from build123d import *

# Parameters (mm, degrees)
REVOLVE_THIN1_ANGLE = 60
SKETCH3_R           = 45
BOSS_EXTRUDE2_DEPTH = 648.5
SKETCH4_R           = 28
CUT_EXTRUDE1_DEPTH  = 40
CUT_EXTRUDE2_DEPTH  = 40


# Read off the part's stored shape, not the designer's step: Revolve-Thin1
with BuildPart() as part:
    # Revolve-Thin1 outline → Revolve-Thin1 (revolve)
    with BuildSketch(Plane(origin=(-45, 0, 0), x_dir=(1, 0, 0), z_dir=(0, 0, 1))):
        with BuildLine():
            Line((35, -19.5), (0, -19.5))
            Line((0, -19.5), (0, -29.5))
            Line((0, -29.5), (45, -29.5))
            Line((45, -29.5), (45, -9.5))
            ThreePointArc((45, -9.5), (54.5, 0), (45, 9.5))
            Line((45, 9.5), (45, 619))
            Line((45, 619), (0, 619))
            Line((0, 619), (0, 609))
            Line((0, 609), (35, 609))
            Line((35, 609), (35, -19.5))
        make_face()
    revolve(axis=Axis((-45, 0, 0), (0, 1, 0)), revolution_arc=REVOLVE_THIN1_ANGLE)

    # Sketch3 → Boss-Extrude2 (add)
    with BuildSketch(Plane(origin=(0, 619, 0), x_dir=(1, 0, 0), z_dir=(0, 1, 0))):
        with Locations(Location((-45, 0, 0), (0, 0, 90))):
            Circle(SKETCH3_R)
    extrude(amount=-BOSS_EXTRUDE2_DEPTH)

    # Sketch4 → Cut-Extrude1 (cut)
    with BuildSketch(Plane(origin=(0, 619, 0), x_dir=(1, 0, 0), z_dir=(0, 1, 0))):
        with Locations(Location((-45, 0, 0), (0, 0, 270))):
            Circle(SKETCH4_R)
    extrude(amount=-CUT_EXTRUDE1_DEPTH, mode=Mode.SUBTRACT)

    # Sketch5 → Cut-Extrude2 (cut)
    with BuildSketch(Plane(origin=(0, 619, 0), x_dir=(1, 0, 0), z_dir=(0, 1, 0))):
        with BuildLine():
            Line((-18.321356856, 8.5), (-12, 8.5))
            Line((-12, 8.5), (-12, -8.5))
            Line((-12, -8.5), (-18.321356856, -8.5))
            ThreePointArc((-18.321356856, -8.5), (-17, 0), (-18.321356856, 8.5))
        make_face()
    extrude(amount=-CUT_EXTRUDE2_DEPTH, mode=Mode.SUBTRACT)


solid = part.part
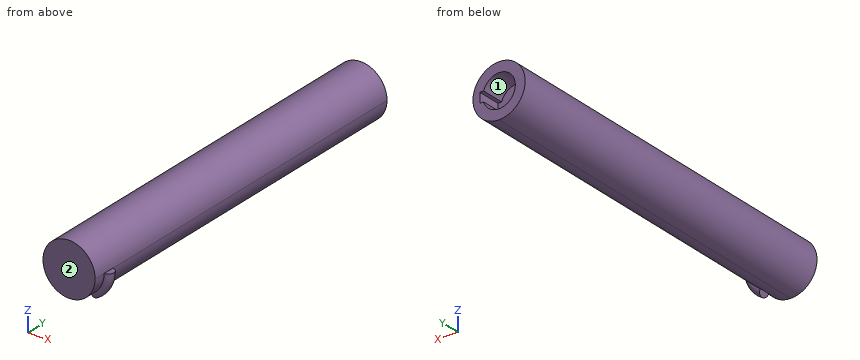
Input: part model. Units: mm. Frame: model coordinates. Face numbers are marked on the shaded views. Give positions to 0.01 mm unless a question says otherwise; leave off trailing zeros. Loops run counter-clockwise (first coordinate to the right, second up) from the corner with the lowest first, then second, coordinate; pieces in that order, holes last. Notation, with made-up numbers: M -12.75,75.5 L 1.25,75.5 A28 cw 1.25,93.5 Z; hole C -20,56.5 d9. An arc over 180 degrees is marked long. Use one line per item in the form item = value.
1. Section query D-D, the plane x = -81. Return the cut outline in (y, z), and give its area (3 significant figures).
Numbers:
outline = M -29.5,-27 L 619,-27 L 619,27 L -29.5,27 Z
area = 35,000 mm²
2. Section query C-C, the plane y = 246. Return the cut outline in (x, z).
Numbers:
outline = C -45,0 d90
3. Line query: L1, parallel to X at y = 609, z = 0; L2, parallel to Y at x = -48.5, z = 11; L3, parallel to X at y = 2, z = 26.5. Output: solid intervals per line, ascending.
Numbers:
L1 = -90 to -73, -12 to 0
L2 = -29.5 to 579
L3 = -81.37 to -8.63
4. Pull-direction query (Z, two-part tool) for the marked faces 1 and 2; classes: released by +Z, released by -Z, zero draft, split by the parting line, or undercut.
Numbers:
face_1 = undercut
face_2 = zero draft
5. First-contact query: pin 1 (2 mm diameter, centred on x = -72, y = 443, fed in from +Z); pin 2 (1 mm diameter, centred on x = -60, y = 423.5, fed in from -Z); pin 3 (12 mm diameter, centred on y = 202, z = -10.5, fed in from -X). Flat tips, straight axial feed; report the tip coordinate or a pass-through.
Numbers:
pin_1 = 36.73
pin_2 = -42.6
pin_3 = -89.77
6. Section query A-A, the plane z = 18. Return the cut outline in (x, y).
Numbers:
outline = M -86.24,-29.5 L -3.76,-29.5 L -3.76,619 L -23.55,619 L -23.55,579 L -66.45,579 L -66.45,619 L -86.24,619 Z
7. Section query B-B, the plane x = -28. Return the cut outline in (y, z), and give its area (3 significant figures).
Numbers:
outline = M -29.5,-41.67 L 619,-41.67 L 619,-22.25 L 579,-22.25 L 579,22.25 L 619,22.25 L 619,41.67 L -29.5,41.67 Z
area = 52,300 mm²
